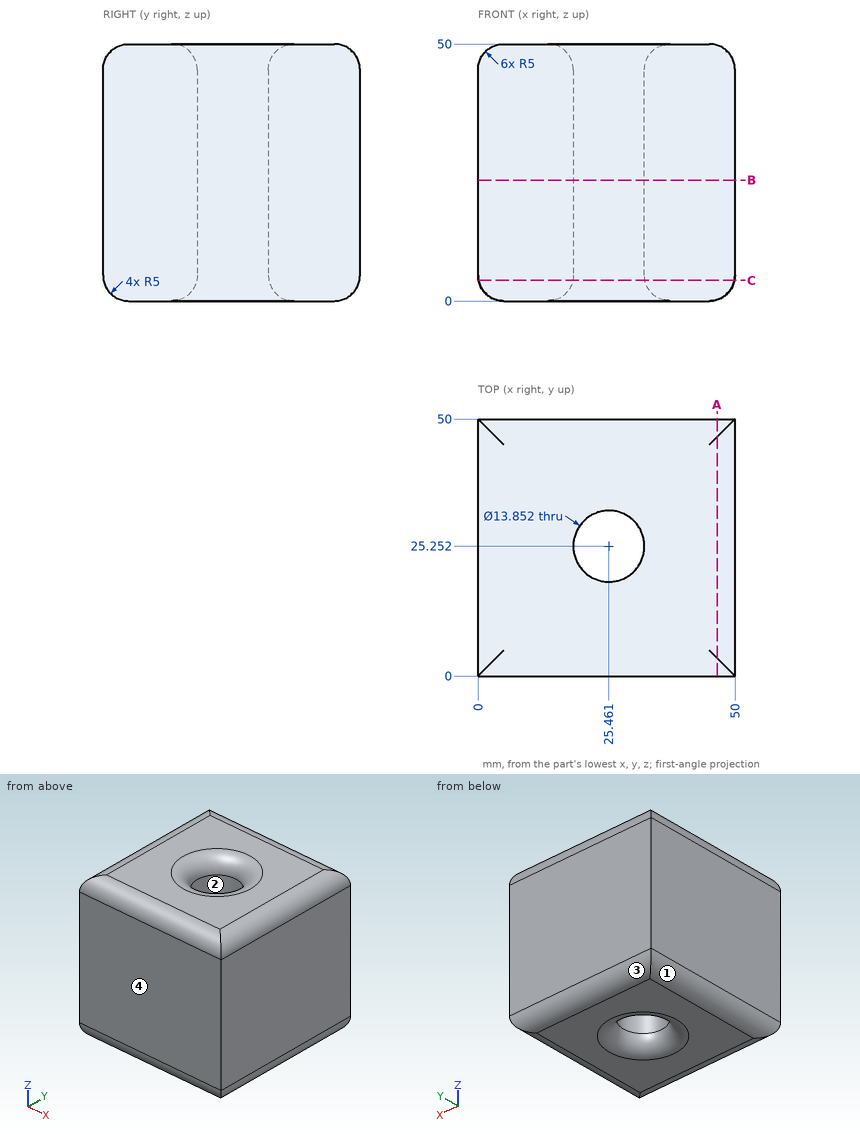
Could you check a few things on this drawing? It's one solid part, dimensions in mm from its lowest x, y, z. Round coordinates to 2 decimals unless told otherwise and drop trailing zeros. Loops run counter-clockwise (first coordinate to the right, second up) from the corner with the lowest first, then second, coordinate; pieces in that order, holes last. Notation, with made-up numbers: (44, 84.25) -> (77, 84.25) arc R29 cw to (77, 111.25) -> close; hole circle Ø1 at (26, -38). An arc over 180 degrees is marked (long way). Answer as CSV lines item,"result".
1. Thinking about a two-plate mould opening in Y: for the marked faces 1, 2, 3 and 4, which applies, released by +Y, released by -Y, zero draft, split by the parting line, or undercut?
Final values:
face 1,"zero draft"
face 2,"undercut"
face 3,"released by +Y"
face 4,"released by -Y"
2. If we section it at C-C on z = 4: Please give me the cut outline in (x, y) (1 decimal), plus the area to 3 significant figures.
Final values:
outline,"(0.1, 0.1) -> (49.9, 0.1) -> (49.9, 49.9) -> (0.1, 49.9) -> close; hole circle Ø14.1 at (25.5, 25.3)"
area,"2,320 mm^2"
3. If we section it at A-A on x = 46.5: Please give me the cut outline in (y, z).
Final values:
outline,"(0, 5) arc R5 ccw to (3.5, 0.23) -> (46.5, 0.23) arc R5 ccw to (50, 5) -> (50, 45) arc R5 ccw to (46.5, 49.77) -> (3.5, 49.77) arc R5 ccw to (0, 45) -> close"
4. If we section it at B-B on z = 23.5: Please give me the cut outline in (x, y).
Final values:
outline,"(0, 0) -> (50, 0) -> (50, 50) -> (0, 50) -> close; hole circle Ø13.85 at (25.46, 25.25)"
5. If I drill on L1, parallel to Y at x = 31, z = 3.5 (1 decimal); L2, parallel to Y at x = 27, z = 30.5 (1 decimal); L3, parallel to X at y = 20, z = 23 (1 decimal), over which ranges is the centre line in solid material (lowest first)?
Final values:
L1,"y = 0.2 to 20.7, 29.8 to 49.8"
L2,"y = 0 to 18.5, 32 to 50"
L3,"x = 0 to 20.9, 30 to 50"
